Read the model definition and answer for the solid it produces. Units are mm, in the model's axes. A direction names the side the tool comes from. Round coordinates to 2 decimals unless told otherwise and drop trailing zeros. Loops run counter-clockwise (first coordinate to the right, second up) from the corner with the lowest first, then second, coordinate; pieces in that order, holes last. Notation, with made-up numbers: (-31, -13.5) - (-4, -13.5) arc R26 ccw to (-4, 18.5) - close; hole circle Ø1 at (42, -17). An arc over 180 degrees is marked (long way). Answer as CSV lines item,"result".
```python
from build123d import *

# Parameters (mm, degrees)
SKETCH_2_W          = 60
SKETCH_2_H          = 68
EXTRUDE_1_DEPTH     = 4
CUT_EXTRUDE_1_DEPTH = 4
SKETCH_4_R          = 1
CUT_EXTRUDE_2_DEPTH = 4


with BuildPart() as part:
    # Эскиз2 → Бобышка-Вытянуть1 (new body)
    with BuildSketch(Plane.XY):
        with Locations((30, 34)):
            Rectangle(SKETCH_2_W, SKETCH_2_H)
    extrude(amount=EXTRUDE_1_DEPTH)

    # Эскиз3 → Вырез-Вытянуть1 (cut)
    with BuildSketch(Plane.XY.offset(4)):
        Polygon((8.65, 0), (8.65, 5.25), (7.4, 5.25), (7.4, 7.75), (8.65, 7.75), (8.65, 13), (11.65, 13), (11.65, 7.75), (12.9, 7.75), (12.9, 5.25), (11.65, 5.25), (11.65, 0), align=None)
        Polygon((47.1, 7.75), (48.35, 7.75), (48.35, 13), (51.35, 13), (51.35, 7.75), (52.6, 7.75), (52.6, 5.25), (51.35, 5.25), (51.35, 0), (48.35, 0), (48.35, 5.25), (47.1, 5.25), align=None)
        Polygon((48.35, 68), (48.35, 62.75), (47.1, 62.75), (47.1, 60.25), (48.35, 60.25), (48.35, 55), (51.35, 55), (51.35, 60.25), (52.6, 60.25), (52.6, 62.75), (51.35, 62.75), (51.35, 68), align=None)
        Polygon((8.65, 68), (8.65, 62.75), (7.4, 62.75), (7.4, 60.25), (8.65, 60.25), (8.65, 55), (11.65, 55), (11.65, 60.25), (12.9, 60.25), (12.9, 62.75), (11.65, 62.75), (11.65, 68), align=None)
    extrude(amount=-CUT_EXTRUDE_1_DEPTH, mode=Mode.SUBTRACT)

    # Эскиз4 → Вырез-Вытянуть2 (cut)
    with BuildSketch(Plane.XY.offset(4)):
        with Locations((2.5, 34)):
            Circle(SKETCH_4_R)
        with Locations((7.5, 34)):
            Circle(SKETCH_4_R)
        with Locations((12.5, 34)):
            Circle(SKETCH_4_R)
        with Locations((17.5, 34)):
            Circle(SKETCH_4_R)
        with Locations((22.5, 34)):
            Circle(SKETCH_4_R)
        with Locations((27.5, 34)):
            Circle(SKETCH_4_R)
        with Locations((32.5, 34)):
            Circle(SKETCH_4_R)
        with Locations((37.5, 34)):
            Circle(SKETCH_4_R)
        with Locations((42.5, 34)):
            Circle(SKETCH_4_R)
        with Locations((47.5, 34)):
            Circle(SKETCH_4_R)
        with Locations((52.5, 34)):
            Circle(SKETCH_4_R)
        with Locations((57.5, 34)):
            Circle(SKETCH_4_R)
    extrude(amount=-CUT_EXTRUDE_2_DEPTH, mode=Mode.SUBTRACT)


solid = part.part
```
1) Find the intervals of material crossed by line 1 (X direction, y = 58.5, z = 0.3); line 2 (Y direction, x = 7.5, z = 1.7); line 3 (X direction, y = 62.5, z = 1.35), in increasing order.
Entries:
line 1,"x = 0 to 8.65, 11.65 to 48.35, 51.35 to 60"
line 2,"y = 0 to 5.25, 7.75 to 33, 35 to 60.25, 62.75 to 68"
line 3,"x = 0 to 7.4, 12.9 to 47.1, 52.6 to 60"
2) A cutting plane is placed at B-B, the plane y = 10. Determine the outline of the cut face in (x, z).
Entries:
outline,"(0, 0) - (8.65, 0) - (8.65, 4) - (0, 4) - close; (11.65, 0) - (48.35, 0) - (48.35, 4) - (11.65, 4) - close; (51.35, 0) - (60, 0) - (60, 4) - (51.35, 4) - close"
3) A cutting plane is placed at A-A, the plane x = 42.5. Determine the outline of the cut face in (y, z), plus the area to 3 significant figures.
Entries:
outline,"(0, 0) - (33, 0) - (33, 4) - (0, 4) - close; (35, 0) - (68, 0) - (68, 4) - (35, 4) - close"
area,"264 mm^2"
4) A cutting plane is placed at C-C, the plane z = 2.5. Count the separate pieces of the cut face and the enclosed holes in it, plus the area to 3 significant figures.
Entries:
separate pieces,"1"
enclosed holes,"12"
area,"3,860 mm^2"
5) The mould has two halves that part along X. Classify faces 4 (the face through (4, 0, 2)), 5 (the face through (52.37, 34.99, 2.03)), 6 (the face through (0, 34, 2)): pulls with the +X half, pulls with the -X half, needs draft (parallel to the pull), parting line crosses it, or undercut.
Entries:
face 4,"needs draft"
face 5,"undercut"
face 6,"pulls with the -X half"
6) A tool of negligible diameter and unlimited length cuts with its end or side. For faces 1 (the face through (10, 55, 2)), 2 (the face through (47.1, 62, 2)), 3 (the face through (8.65, 10, 2)), from which of +Z, -Z, +X, -X, +Y, -Y can it reach the whole face along a straight path? Write none if from no direction.
Entries:
face 1,"+Z, -Z, +Y"
face 2,"+Z, -Z"
face 3,"+Z, -Z, -Y"
7) This flat-tipped pin is pushed along its axis until it touches: P1, Ø4, axis at x = 12, y = 11, coming from the -Z side. Where does it stop, or does it pass through?
Entries:
P1,"stops at z = 0"
